Can you work these out from the model? Positions are in its coordinate system, mm. A direction names the side the tool comes from. Coordinates: 2 decimals unless noted, no trailing zeros. Write each loop counter-clockwise with the first axis right and the second up, starting at its lowest first coordinate (ties: lowest second). Pieces come first, ordered by that corner, then holes. Notation, with made-up numbers: M 43,-38 L 62,-38 A31 ccw 62,-13 Z; hole C -16,-27 d1. An arc over 180 degrees is marked long. Use one line per item in the form item = value. Start each with the question number.
```python
from build123d import *
from build123d import SkipClean  # not in build123d's __all__


with BuildPart() as f1:
    # F0 (on Front) → F1 (revolve)
    with BuildSketch(Plane.XZ):
        Polygon((0, 19.05), (-12.7, 19.05), (-12.7, 0), (0, 0), (50.8, 0), (50.8, 12.573), (0, 12.573), align=None)
    revolve(axis=Axis((25.4, 0, 0), (1, 0, 0)))

    # F2 (on Front) → F3 (revolve, cut)
    with BuildSketch(Plane.XZ):
        with BuildLine():
            Line((57.15, 0), (57.15, 12.573))
            ThreePointArc((57.15, 12.573), (44.577, 0), (57.15, -12.573))
            Line((57.15, -12.573), (57.15, 0))
        make_face()
    with SkipClean():  # cleaning this boolean's faces spoils the solid; the shape is the same uncleaned
        revolve(axis=Axis((57.15, 0, 0), (0, 0, 1)), mode=Mode.SUBTRACT)


solid = f1.part
```
1) Which directions (+Z, -Z, +X, -X, +Y, -Y) give clear straight access to the entire face, cutting with the end or side of a thin tool? Please do faces 1 (the face through (25.044, 12.274, -2.726)), 2 (the face through (-12.7, 0, 0)).
2) Will these pins go through, and if not, where does the flat tip stop? pin 1 Ø2 at (x, y) = (19, 8.5) entering from +Z; pin 2 Ø3 at (x, y) = (6, 7.5) entering from +Z; pin 3 Ø1.5 at (y, z) = (-14.5, -4.5) entering from +X; pin 4 Ø1.5 at (x, y) = (14, 14) entering from -Z (1 decimal).
3) Suppose I cut it at D-D on x = -5. Please give me the cut outline in (y, z).
4) Please list where these lines run through material, in increasing order: line 1 (X direction, y = 5, z = -15.5); line 2 (Y direction, x = 22, z = 0).
5) Suppose I cut it at A-A on x = 35.5. Please give me the cut outline in (y, z).
6) Suppose I cut it at B-B on z = 14. Please give me the cut outline in (x, y).
7) Suppose I cut it at C-C on y = 16.5. Please give me the cut outline in (x, z), and give its area (3 significant figures).
Computed values:
q1.face_1 = +X
q1.face_2 = +Z, -Z, -X, +Y, -Y
q2.pin_1 = 10.09
q2.pin_2 = 11.05
q2.pin_3 = 0
q2.pin_4 = through
q3.outline = C 0,0 d38.1
q4.line_1 = -12.7 to 0
q4.line_2 = -12.57 to 12.57
q5.outline = C 0,0 d25.15
q6.outline = M -12.7,-12.92 L 0,-12.92 L 0,12.92 L -12.7,12.92 Z
q7.outline = M -12.7,-9.52 L 0,-9.52 L 0,9.52 L -12.7,9.52 Z
q7.area = 242 mm²
